Can you work these out from the model? Positions are in its coordinate system, mm. A direction names the side the tool comes from. Round coordinates to 2 decimals unless told otherwise and drop trailing zeros. Loops run counter-clockwise (first coordinate to the right, second up) from the corner with the lowest first, then second, coordinate; pieces in that order, holes last. Notation, with made-up numbers: M 79,2 L 86,2 A29 cw 86,37 Z; hole C 33,27 d5. An arc over 180 degrees is marked long. Use a Markdown table: item, result. Add a question column.
```python
from build123d import *

# Parameters (mm, degrees)
EXTRUDE1_DEPTH        = 30
FILLET1_R             = 5
M5_TAPPED_HOLE1_D     = 4.2
M6_TAPPED_HOLE1_D     = 5
M6_TAPPED_HOLE1_DEPTH = 20
M6_TAPPED_HOLE1_TIP   = 1.502151548


with BuildPart() as part:
    # Sketch1 → Extrude1 (new body)
    with BuildSketch(Plane.XY):
        with BuildLine():
            Line((-25, 31.5), (25, 31.5))
            Line((25, 31.5), (25, -20))
            Line((25, -20), (8.5, -20))
            Line((8.5, -20), (8.5, -11.124297731))
            ThreePointArc((8.5, -11.124297731), (0, 14), (-8.5, -11.124297731))
            Line((-8.5, -11.124297731), (-8.5, -20))
            Line((-8.5, -20), (-25, -20))
            Line((-25, -20), (-25, 31.5))
        make_face()
    extrude(amount=EXTRUDE1_DEPTH)

    # Fillet1
    fillet1_edges = [part.edges().sort_by_distance(p)[0] for p in [
        (-8.5, -20, 15),
        (-25, -20, 15),
        (25, -20, 15),
        (8.5, -20, 15),
        (8.5, -11.124297731, 15),
        (-8.5, -11.124297731, 15),
    ]]
    fillet(fillet1_edges, radius=FILLET1_R)

    # M5 Tapped Hole1 (through all)
    with Locations(Plane(origin=(0, 0, 0), x_dir=(-1, 0, 0), z_dir=(0, 0, -1))):
        with Locations((-13.435028843, 13.435028843), (13.435028843, 13.435028843), (19, 0), (13.435028843, -13.435028843), (-13.435028843, -13.435028843), (-19, 0)):
            Hole(M5_TAPPED_HOLE1_D / 2)

    # M6 Tapped Hole1
    with Locations(Plane(origin=(0, 31.5, 0), x_dir=(1, 0, 0), z_dir=(0, 1, 0))):
        with Locations((-17.5, -15), (17.5, -15)):
            Hole(M6_TAPPED_HOLE1_D / 2, depth=M6_TAPPED_HOLE1_DEPTH)
            with Locations((0, 0, -(M6_TAPPED_HOLE1_DEPTH + M6_TAPPED_HOLE1_TIP / 2))):  # 118° drill point
                Cone(0, M6_TAPPED_HOLE1_D / 2, M6_TAPPED_HOLE1_TIP, mode=Mode.SUBTRACT)


solid = part.part
```
(1) I'm going to push flat-ended pins straight in: pin 1 (5 mm diameter, centred on x = -14.5, y = 7, fed in from -Z); pin 2 (6 mm diameter, centred on x = -4, z = 19.5, fed in from -Y); pin 3 (3 mm diameter, centred on x = -17.5, z = 15, fed in from +Y). Where does each tip first touch, or does it pass through?
(2) If I drill on probe 1 along Y at (x, z) = (15, 13.5); probe 2 along Z at (x, y) = (17.5, 25.75); probe 3 along X at (y, z) = (-13, 3), over which ranges is the centre line in solid material (lowest first)? Write a range as [from, to].
(3) On a 3-axis mill with a long thin cutter (end or side, diameter ignored), from which of +Z, -Z, +X, -X, +Y, -Y can I reach the whole of each face in a straight line? I mean faces 1 (the face through (10, -18.57, 15.21)), 2 (the face through (24, -18, 15)), 3 (the face through (-19.81, 21.36, 15.96)). Say none if no direction works.
(4) Suppose I cut it at A-A on y = 0. List the corners of the cut face in (x, z) for me, and give its area (3 significant figures).
(5) Suppose I cut it at B-B on z = 24. List the corners of the cut face in (x, y) for me, and give its area (3 significant figures).
(6) Thinking about a two-plate mould opening in X: for faces 4 (the face through (25, 9, 15)), 5 (the face through (20, 21, 15)), 6 (the face through (0, 18, 30)), which applies, released by +X, released by -X, zero draft, split by the parting line, or undercut?
(7) Suppose I cut it at C-C on x = 0. List the corners of the cut face in (y, z) for me, and give its area (3 significant figures).
Results below:
| question | item | result |
|---|---|---|
| 1 | pin 1 | stops at z = 0 |
| 1 | pin 2 | stops at y = 12.12 |
| 1 | pin 3 | stops at y = 10.9 |
| 2 | probe 1 | y = [-20, -14.84], [-12.03, 12.03], [14.84, 31.5] |
| 2 | probe 2 | z = [0, 12.5], [17.5, 30] |
| 2 | probe 3 | x = [-25, -15.49], [-11.38, -8.51], [8.51, 11.38], [15.49, 25] |
| 3 | face 1 | +Z, -Z, -Y |
| 3 | face 2 | +Z, -Z, +X, -Y |
| 3 | face 3 | +Y |
| 4 | outline | M -25,0 L -21.1,0 L -21.1,30 L -25,30 Z; M -16.9,0 L -14,0 L -14,30 L -16.9,30 Z; M 14,0 L 16.9,0 L 16.9,30 L 14,30 Z; M 21.1,0 L 25,0 L 25,30 L 21.1,30 Z |
| 4 | area | 408 mm² |
| 5 | outline | M -25,-15 A5 ccw -20,-20 L -13.5,-20 A5 ccw -8.5,-15 L -8.5,-13.37 A5 ccw -9.95,-9.85 A14 cw long 9.95,-9.85 A5 ccw 8.5,-13.37 L 8.5,-15 A5 ccw 13.5,-20 L 20,-20 A5 ccw 25,-15 L 25,31.5 L -25,31.5 Z; hole C -19,0 d4.2; hole C -13.44,-13.44 d4.2; hole C -13.44,13.44 d4.2; hole C 13.44,-13.44 d4.2; hole C 13.44,13.44 d4.2; hole C 19,0 d4.2 |
| 5 | area | 1,740 mm² |
| 6 | face 4 | released by +X |
| 6 | face 5 | undercut |
| 6 | face 6 | zero draft |
| 7 | outline | M 14,0 L 31.5,0 L 31.5,30 L 14,30 Z |
| 7 | area | 525 mm² |
